from build123d import *

# Parameters (mm, degrees)
SKETCH2_R           = 4.2
BOSS_EXTRUDE1_DEPTH = 1.2
SKETCH3_R           = 3
BOSS_EXTRUDE2_DEPTH = 4.3
SKETCH4_OUTSIDE_W   = 14.534
SKETCH4_OUTSIDE_H   = 14.534
SKETCH4_OUTSIDE_R   = 2.8
CUT_EXTRUDE1_DEPTH  = 4.3
CUT_EXTRUDE1_TAPER  = 10
SKETCH5_R           = 2
CUT_EXTRUDE2_DEPTH  = 6.5


with BuildPart() as part:
    # Sketch2 → Boss-Extrude1 (new body)
    with BuildSketch(Plane(origin=(0, 0, 0), x_dir=(1, 0, 0), z_dir=(0, 1, 0))):
        Circle(SKETCH2_R)
    extrude(amount=BOSS_EXTRUDE1_DEPTH)

    # Sketch3 → Boss-Extrude2 (add)
    with BuildSketch(Plane(origin=(0, 1.2, 0), x_dir=(1, 0, 0), z_dir=(0, 1, 0))):
        Circle(SKETCH3_R)
    extrude(amount=BOSS_EXTRUDE2_DEPTH)

    # Sketch4 outside → Cut-Extrude1 (cut)
    with BuildSketch(Plane(origin=(0, 5.5, 0), x_dir=(1, 0, 0), z_dir=(0, 1, 0))):
        Rectangle(SKETCH4_OUTSIDE_W, SKETCH4_OUTSIDE_H)
        Circle(SKETCH4_OUTSIDE_R, mode=Mode.SUBTRACT)
    extrude(amount=-CUT_EXTRUDE1_DEPTH, taper=CUT_EXTRUDE1_TAPER, mode=Mode.SUBTRACT)

    # Sketch5 → Cut-Extrude2 (cut, through all)
    with BuildSketch(Plane(origin=(0, 5.5, 0), x_dir=(1, 0, 0), z_dir=(0, 1, 0))):
        Circle(SKETCH5_R)
    extrude(amount=-CUT_EXTRUDE2_DEPTH, mode=Mode.SUBTRACT)


solid = part.part
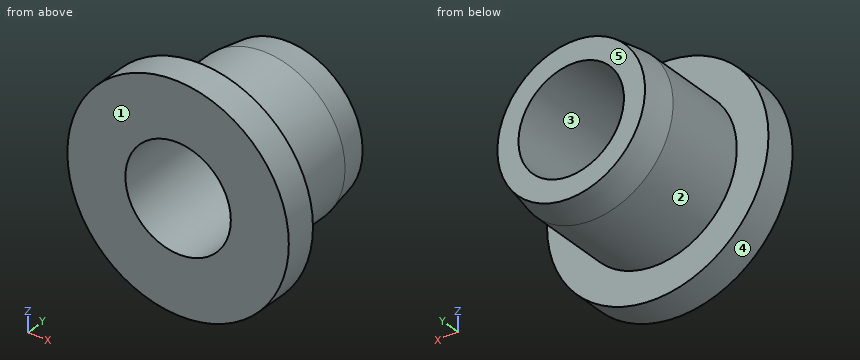
Build history of the part. All positions in model axes, mm. Face numbers are marked on the shaded views. A direction names the side the tool comes from. Coordinates: 2 decimals unless noted, no trailing zeros. Write each loop counter-clockwise with the first axis right and the second up, starting at its lowest first coordinate (ties: lowest second). Pieces come first, ordered by that corner, then holes. Notation, with made-up numbers: (41.25, -32.5) -> (93.25, -32.5) arc R15 cw to (93.25, -6.5) -> close; hole circle Ø3 at (85, -20.5). An arc over 180 degrees is marked (long way). Use CSV: the item, a comma, the result in double quotes. Start each with the question number.
Q1. Flat gauge pin, fed straight in: pin 1 Ø1.5 at (x, y) = (-1, 4.5) entering from +Z. Where does the tip first touch, or does it go through?
Q2. 3-axis set-ups, long thin cutter, end or side, ignore diameter. For the marked faces 1 and 2: which of +Z, -Z, +X, -X, +Y, -Y reach the whole face in a straight line?
Q3. Cut at D-D, the plane z = 3.75. List the corners of the cut face in (x, y).
Q4. Pull direction Z, two halves, no side cores. Call the marked faces 3, 4 and 5: released by +Z, released by -Z, zero draft, split by the parting line, or undercut.
Q5. Cut at B-B, the plane y = 0.85. List the corners of the cut face in (x, z), then the cut area to 3 significant figures.
Q6. Drill centre lines: probe 1 along X at (y, z) = (2.3, 0); probe 2 along X at (y, z) = (5.2, 1.25). Where is each one in solid material? Low to high.
Q7. Cut at A-A, the plane x = 0. List the corners of the cut face in (y, z), then the cut area to 3 significant figures.
Q8. Cut at C-C, the plane y = 2.25. List the corners of the cut face in (x, z).
Checked values:
1,pin 1,"stops at z = 2.99"
2,face 1,"+Z, -Z, +X, -X, -Y"
2,face 2,"+Y"
3,outline,"(-1.89, 0) -> (1.89, 0) -> (1.89, 1.2) -> (-1.89, 1.2) -> close"
4,face 3,"undercut"
4,face 4,"split by the parting line"
4,face 5,"zero draft"
5,outline,"circle Ø8.4 at (0, 0); hole circle Ø4 at (0, 0)"
5,area,"42.9 mm²"
6,probe 1,"x = -3 to -2, 2 to 3"
6,probe 2,"x = -2.56 to -1.56, 1.56 to 2.56"
7,outline,"(0, -4.2) -> (1.2, -4.2) -> (1.2, -3) -> (4.37, -3) -> (5.5, -2.8) -> (5.5, -2) -> (0, -2) -> close; (0, 2) -> (5.5, 2) -> (5.5, 2.8) -> (4.37, 3) -> (1.2, 3) -> (1.2, 4.2) -> (0, 4.2) -> close"
7,area,"13.7 mm²"
8,outline,"circle Ø6 at (0, 0); hole circle Ø4 at (0, 0)"
